```python
from build123d import *

# Parameters (mm, degrees)
BLOCK_SKETCH_W      = 14.3
BLOCK_SKETCH_H      = 14.3
BLOCK_DEPTH         = 7.15
ARM_X_SKETCH_W      = 19.75
ARM_X_SKETCH_H      = 7.722
ARM_Y_SKETCH_W      = 7.722
ARM_Y_SKETCH_H      = 19.75
SOCKET_X_SKETCH_W   = 16.2
SOCKET_X_SKETCH_H   = 3.175
SOCKET_Y_SKETCH_W   = 3.175
SOCKET_Y_SKETCH_H   = 16.2
ARM_X_SKETCH_2_W    = 19.75
ARM_X_SKETCH_2_H    = 7.722
SOCKET_X_SKETCH_2_W = 16.2
SOCKET_X_SKETCH_2_H = 3.175


with BuildPart() as part:
    # Block Sketch → Block (new, symmetric)
    with BuildSketch(Plane.XY):
        Rectangle(BLOCK_SKETCH_W, BLOCK_SKETCH_H)
    extrude(amount=BLOCK_DEPTH, both=True)

    # Arm X Sketch → Arm X (revolve)
    with BuildSketch(Plane.XY, mode=Mode.PRIVATE) as arm_x_sk:
        with Locations((17.025, 3.861)):
            Rectangle(ARM_X_SKETCH_W, ARM_X_SKETCH_H)
    revolve(arm_x_sk.sketch.rotate(Axis((-1000, 0, 0), (1, 0, 0)), 90), axis=Axis((-1000, 0, 0), (1, 0, 0)))

    # Arm Y Sketch → Arm Y (revolve)
    with BuildSketch(Plane.XY, mode=Mode.PRIVATE) as arm_y_sk:
        with Locations((3.861, 17.025)):
            Rectangle(ARM_Y_SKETCH_W, ARM_Y_SKETCH_H)
    revolve(arm_y_sk.sketch.rotate(Axis((0, -500, 0), (0, 1, 0)), 90), axis=Axis((0, -500, 0), (0, 1, 0)))

    # Socket X Sketch → Socket X (revolve, cut)
    with BuildSketch(Plane.XY, mode=Mode.PRIVATE) as socket_x_sk:
        with Locations((19.8, 1.5875)):
            Rectangle(SOCKET_X_SKETCH_W, SOCKET_X_SKETCH_H)
    revolve(socket_x_sk.sketch.rotate(Axis((-1000, 0, 0), (1, 0, 0)), 90), axis=Axis((-1000, 0, 0), (1, 0, 0)), mode=Mode.SUBTRACT)

    # Socket Y Sketch → Socket Y (revolve, cut)
    with BuildSketch(Plane.XY, mode=Mode.PRIVATE) as socket_y_sk:
        with Locations((1.5875, 19.8)):
            Rectangle(SOCKET_Y_SKETCH_W, SOCKET_Y_SKETCH_H)
    revolve(socket_y_sk.sketch.rotate(Axis((0, -500, 0), (0, 1, 0)), 90), axis=Axis((0, -500, 0), (0, 1, 0)), mode=Mode.SUBTRACT)

    # Arm -X Sketch 2 → Arm -X 2 (revolve)
    with BuildSketch(Plane.XY, mode=Mode.PRIVATE) as arm_x_2_sk:
        with Locations((-17.025, 3.861)):
            Rectangle(ARM_X_SKETCH_2_W, ARM_X_SKETCH_2_H)
    revolve(arm_x_2_sk.sketch.rotate(Axis((-1000, 0, 0), (1, 0, 0)), 90), axis=Axis((-1000, 0, 0), (1, 0, 0)))

    # Socket -X Sketch 2 → Socket -X 2 (revolve, cut)
    with BuildSketch(Plane.XY, mode=Mode.PRIVATE) as socket_x_2_sk:
        with Locations((-19.8, 1.5875)):
            Rectangle(SOCKET_X_SKETCH_2_W, SOCKET_X_SKETCH_2_H)
    revolve(socket_x_2_sk.sketch.rotate(Axis((-1000, 0, 0), (1, 0, 0)), 90), axis=Axis((-1000, 0, 0), (1, 0, 0)), mode=Mode.SUBTRACT)


solid = part.part
```
Work out the finished part from the listing and answer in its coordinate system (mm). A direction names the side the tool comes from. Give positions to 0.01 mm unless a question says otherwise; leave off trailing zeros. Loops run counter-clockwise (first coordinate to the right, second up) from the corner with the lowest first, then second, coordinate; pieces in that order, holes last. Notation, with made-up numbers: (51.5, 44.25) -> (56.5, 44.25) arc R24 cw to (56.5, 55.25) -> close; hole circle Ø9 at (-0.75, -14.5). An arc over 180 degrees is marked (long way). Write item = value, one per line. Start each with the question number.
(1) Find section A-A on y = 0. Give the vertices of the cut face in (x, z) (3 decimals), and give its area (3 significant figures).
(2) The mould has two halves that part along Y. Classify faces 6 (the flat face through (6, 7.15, -6)), 7 (the flat face through (-7.15, 6, 6)), 8 (the flat face through (11.7, 0, 0)), 9 (the cylindrical face through (-19.19, 1.93, -2.52)): +Y half, -Y half, draft (parallel to the pull), parting line (faces both ways), or undercut.
(3) Find section C-C on x = 0. Give the vertices of the cut face in (y, z) (3 decimals).
(4) Which of the six approach directions +Z, -Z, +X, -X, +Y, -Y give full straight-line access (tool end or side, diameter ignored) to faces 1 (the flat face through (0, 0, 7.15)), 2 (the cylindrical face through (-16.887, -7.656, -1.005)), 3 (the flat face through (7.15, 6, 6)), 4 (the flat face through (-7.15, -6, 6)), 5 (the flat face through (7.15, 6, -6))?
(5) Given pin 1 Ø3 at (y, z) = (0, 0) entering from +X; pin 2 Ø2 at (x, z) = (-9, 3.5) entering from +Y; pin 3 Ø1.9 at (y, z) = (-1, 0) entering from -X, each flat-ended and moving along its own axis, determine where each tip first touches the part or whether it passes through.
(6) Find the intervals of material crossed by probe 1 along Y at (x, z) = (17.75, 0) (3 decimals); probe 2 along Z at (x, y) = (1.5, -5.5); probe 3 along Y at (x, z) = (-19, 2.75), in increasing order. Write a range as from..to.
(7) Find section D-D on y = 19.5. Give the vertices of the cut face in (x, z) (3 decimals), and give its area (3 significant figures).
(8) Find section B-B on z = 0. Give the vertices of the cut face in (x, y) (3 decimals).
From the geometry:
q1.outline = (-26.9, -7.722) -> (-7.15, -7.722) -> (-7.15, -7.15) -> (7.15, -7.15) -> (7.15, -7.722) -> (26.9, -7.722) -> (26.9, -3.175) -> (11.7, -3.175) -> (11.7, 3.175) -> (26.9, 3.175) -> (26.9, 7.722) -> (7.15, 7.722) -> (7.15, 7.15) -> (-7.15, 7.15) -> (-7.15, 7.722) -> (-26.9, 7.722) -> (-26.9, 3.175) -> (-11.7, 3.175) -> (-11.7, -3.175) -> (-26.9, -3.175) -> close
q1.area = 621 mm^2
q2.face_6 = +Y half
q2.face_7 = draft
q2.face_8 = undercut
q2.face_9 = undercut
q3.outline = (-7.15, -7.15) -> (7.15, -7.15) -> (7.15, -7.722) -> (26.9, -7.722) -> (26.9, -3.175) -> (11.7, -3.175) -> (11.7, 3.175) -> (26.9, 3.175) -> (26.9, 7.722) -> (7.15, 7.722) -> (7.15, 7.15) -> (-7.15, 7.15) -> close
q4.face_1 = +Z, -Y
q4.face_2 = -X
q4.face_3 = +Z, +X, +Y
q4.face_4 = +Z, -X, -Y
q4.face_5 = -Z, +X, +Y
q5.pin_1 = 11.7
q5.pin_2 = 7.31
q5.pin_3 = -11.7
q6.probe_1 = -7.722..-3.175, 3.175..7.722
q6.probe_2 = -7.15..7.15
q6.probe_3 = -7.22..-1.59, 1.59..7.22
q7.outline = circle Ø15.444 at (0, 0); hole circle Ø6.35 at (0, 0)
q7.area = 156 mm^2
q8.outline = (-26.9, -7.722) -> (-7.15, -7.722) -> (-7.15, -7.15) -> (7.15, -7.15) -> (7.15, -7.722) -> (26.9, -7.722) -> (26.9, -3.175) -> (11.7, -3.175) -> (11.7, 3.175) -> (26.9, 3.175) -> (26.9, 7.722) -> (7.722, 7.722) -> (7.722, 26.9) -> (3.175, 26.9) -> (3.175, 11.7) -> (-3.175, 11.7) -> (-3.175, 26.9) -> (-7.722, 26.9) -> (-7.722, 7.722) -> (-26.9, 7.722) -> (-26.9, 3.175) -> (-11.7, 3.175) -> (-11.7, -3.175) -> (-26.9, -3.175) -> close
